from build123d import *

# Parameters (mm, degrees)
PAD_DEPTH       = 2.5
PAD001_DEPTH    = 1
SKETCH003_R     = 1.6
POCKET_DEPTH    = 3.501
SKETCH004_R     = 3.6
SKETCH004_R_2   = 1.6
PAD002_DEPTH    = 2.5
POCKET003_DEPTH = 2.5
CHAMFER005_SIZE = 0.7


with BuildPart() as part:
    # Sketch001 → Pad (new body)
    with BuildSketch(Plane.XY):
        with BuildLine():
            Line((-21.59, 27.9), (11.43, 27.9))
            ThreePointArc((17.74, 21.59), (15.891844, 26.051844), (11.43, 27.9))
            Line((17.74, 21.59), (17.74, -21.59))
            ThreePointArc((11.43, -27.9), (15.891844, -26.051844), (17.74, -21.59))
            Line((11.43, -27.9), (-21.59, -27.9))
            ThreePointArc((-27.9, -21.59), (-26.051844, -26.051844), (-21.59, -27.9))
            Line((-27.9, -21.59), (-27.9, -8.89))
            ThreePointArc((-25.36, -5.326294), (-27.200016, -6.701873), (-27.9, -8.89))
            Line((-25.36, -5.326294), (-25.36, 5.326294))
            ThreePointArc((-27.9, 8.89), (-27.200016, 6.701873), (-25.36, 5.326294))
            Line((-27.9, 8.89), (-27.9, 21.59))
            ThreePointArc((-21.59, 27.9), (-26.051844, 26.051844), (-27.9, 21.59))
        make_face()
        with BuildLine():
            Line((-21.59, 25.9), (11.43, 25.9))
            ThreePointArc((15.74, 21.59), (14.47763, 24.63763), (11.43, 25.9))
            Line((15.74, 21.59), (15.74, -21.59))
            ThreePointArc((11.43, -25.9), (14.47763, -24.63763), (15.74, -21.59))
            Line((11.43, -25.9), (-21.59, -25.9))
            ThreePointArc((-25.9, -21.59), (-24.63763, -24.63763), (-21.59, -25.9))
            Line((-25.9, -21.59), (-25.9, -8.89))
            ThreePointArc((-24.13, -7.12), (-25.381579, -7.638421), (-25.9, -8.89))
            ThreePointArc((-24.13, -7.12), (-23.585528, -6.894472), (-23.36, -6.35))
            Line((-23.36, -6.35), (-23.36, 6.35))
            ThreePointArc((-23.36, 6.35), (-23.585528, 6.894472), (-24.13, 7.12))
            ThreePointArc((-25.9, 8.89), (-25.381579, 7.638421), (-24.13, 7.12))
            Line((-25.9, 8.89), (-25.9, 21.59))
            ThreePointArc((-21.59, 25.9), (-24.63763, 24.63763), (-25.9, 21.59))
        make_face(mode=Mode.SUBTRACT)
    extrude(amount=-PAD_DEPTH)

    # Sketch002 (on Face28 of Pad) → Pad001 (join)
    with BuildSketch(Plane(origin=(0, 0, -2.5), x_dir=(1, 0, 0), z_dir=(0, 0, -1))):
        with BuildLine():
            Line((-21.59, 27.9), (11.43, 27.9))
            ThreePointArc((17.74, 21.59), (15.891844, 26.051844), (11.43, 27.9))
            Line((17.74, 21.59), (17.74, -21.59))
            ThreePointArc((11.43, -27.9), (15.891844, -26.051844), (17.74, -21.59))
            Line((11.43, -27.9), (-21.59, -27.9))
            ThreePointArc((-27.9, -21.59), (-26.051844, -26.051844), (-21.59, -27.9))
            Line((-27.9, -21.59), (-27.9, -8.89))
            ThreePointArc((-25.36, -5.326294), (-27.200016, -6.701873), (-27.9, -8.89))
            Line((-25.36, -5.326294), (-25.36, 5.326294))
            ThreePointArc((-27.9, 8.89), (-27.200016, 6.701873), (-25.36, 5.326294))
            Line((-27.9, 8.89), (-27.9, 21.59))
            ThreePointArc((-21.59, 27.9), (-26.051844, 26.051844), (-27.9, 21.59))
        make_face()
    extrude(amount=PAD001_DEPTH)

    # Sketch003 (on Face31 of Pad001) → Pocket (cut, through all)
    with BuildSketch(Plane(origin=(0, 0, -3.5), x_dir=(1, 0, 0), z_dir=(0, 0, -1))):
        with Locations((-21.59, 21.59)):
            Circle(SKETCH003_R)
        with Locations((11.43, 21.59)):
            Circle(SKETCH003_R)
        with Locations((11.43, -21.59)):
            Circle(SKETCH003_R)
        with Locations((-21.59, -21.59)):
            Circle(SKETCH003_R)
    extrude(amount=-POCKET_DEPTH, mode=Mode.SUBTRACT)

    # Sketch004 (on Face41 of Pocket) → Pad002 (join)
    with BuildSketch(Plane.XY.offset(-2.5)):
        with Locations((11.43, 21.59)):
            Circle(SKETCH004_R)
        with Locations((11.43, 21.59)):
            Circle(SKETCH004_R_2, mode=Mode.SUBTRACT)
        with Locations((-21.59, 21.59)):
            Circle(SKETCH004_R)
        with Locations((-21.59, 21.59)):
            Circle(SKETCH004_R_2, mode=Mode.SUBTRACT)
        with Locations((11.43, -21.59)):
            Circle(SKETCH004_R)
        with Locations((11.43, -21.59)):
            Circle(SKETCH004_R_2, mode=Mode.SUBTRACT)
        with Locations((-21.59, -21.59)):
            Circle(SKETCH004_R)
        with Locations((-21.59, -21.59)):
            Circle(SKETCH004_R_2, mode=Mode.SUBTRACT)
    extrude(amount=PAD002_DEPTH)

    # Sketch012 (on Face31 of Pad002) → Pocket003 (cut)
    with BuildSketch(Plane(origin=(0, 0, -3.5), x_dir=(1, 0, 0), z_dir=(0, 0, -1))):
        Polygon((-18.414574, -21.59), (-20.002287, -18.84), (-23.177713, -18.84), (-24.765426, -21.59), (-23.177713, -24.34), (-20.002287, -24.34), align=None)
        Polygon((8.254574, -21.59), (9.842287, -24.34), (13.017713, -24.34), (14.605426, -21.59), (13.017713, -18.84), (9.842287, -18.84), align=None)
        Polygon((-24.765426, 21.59), (-23.177713, 18.84), (-20.002287, 18.84), (-18.414574, 21.59), (-20.002287, 24.34), (-23.177713, 24.34), align=None)
        Polygon((14.605426, 21.59), (13.017713, 24.34), (9.842287, 24.34), (8.254574, 21.59), (9.842287, 18.84), (13.017713, 18.84), align=None)
    extrude(amount=-POCKET003_DEPTH, mode=Mode.SUBTRACT)

    # Chamfer005
    chamfer005_edges = [part.edges().sort_by_distance(p)[0] for p in [
        (-25.19, 21.59, -2.5),
        (7.83, 21.59, -2.5),
        (-25.19, -21.59, -2.5),
        (7.83, -21.59, -2.5),
    ]]
    chamfer(chamfer005_edges, length=CHAMFER005_SIZE)


solid = part.part
Work out the finished part from the listing and answer in its coordinate system (mm). A direction names the side the tool comes from. Round coordinates to 2 decimals unless told otherwise and drop trailing zeros. Write each loop counter-clockwise with the first axis right and the second up, starting at its lowest first coordinate (ties: lowest second). Pieces come first, ordered by that corner, then holes. Notation, with made-up numbers: (39, 83.25) -> (63, 83.25) arc R12 ccw to (63, 99.25) -> close; hole circle Ø4 at (46, 5). An arc over 180 degrees is marked (long way). Write each question's results on one line, items separated by ' | '.
Item 1: Which of the six approach directions +Z, -Z, +X, -X, +Y, -Y give full straight-line access (tool end or side, diameter ignored) to faces 1 (the face through (-25.9, 15, -1)), 2 (the face through (-27.9, -15, -2)), 3 (the face through (13.82, 20.23, -2.27))?
Result set:
face 1: +Z | face 2: +Z, -Z, -X, +Y, -Y | face 3: -Z
Item 2: Flat-ended cylindrical pins translate along their axes: P1, Ø3.5, axis at x = 11.43, y = 21.59, coming from the +Z side; P2, Ø1, axis at y = 2.5, z = -2, coming from the -X side. Find the tip coordinate at first contact, or state that the pin passes through.
Result set:
P1: z = 0 | P2: x = -25.36
Item 3: The mould has two halves that part along X. Classify faces 4 (the face through (11, 18.84, -2)), 5 (the face through (-27.2, 6.7, -1.7)): +X half, -X half, draft (parallel to the pull), parting line (faces both ways), or undercut.
Result set:
face 4: undercut | face 5: -X half
Item 4: A cutting plane is placed at B-B, the plane x = -4. Determine the outline of the cut face in (y, z), plus the area to 3 significant figures.
Result set:
outline: (-27.9, -3.5) -> (27.9, -3.5) -> (27.9, 0) -> (25.9, 0) -> (25.9, -2.5) -> (-25.9, -2.5) -> (-25.9, 0) -> (-27.9, 0) -> close | area: 65.8 mm^2
Item 5: A cutting plane is placed at A-A, the plane y = 14.5. Determine the outline of the cut face in (x, z).
Result set:
outline: (-27.9, -3.5) -> (17.74, -3.5) -> (17.74, 0) -> (15.74, 0) -> (15.74, -2.5) -> (-25.9, -2.5) -> (-25.9, 0) -> (-27.9, 0) -> close
Item 6: Find the intervals of material crossed by line 1 along Y through (x, z) = (-21.59, -0.4); line 2 along Y through (x, z) = (-9, -1.3); line 3 along Y through (x, z) = (-21.5, -2.15), in increasing order. Write a range as [from, to].
Result set:
line 1: [-27.9, -25.9], [-25.19, -23.19], [-19.99, -17.99], [17.99, 19.99], [23.19, 25.19], [25.9, 27.9] | line 2: [-27.9, -25.9], [25.9, 27.9] | line 3: [-27.9, -25.9], [-25.54, -24.34], [-18.84, -17.64], [17.64, 18.84], [24.34, 25.54], [25.9, 27.9]
